Could you check a few things on this model? Use its own coordinates, in mm. Face numbers are marked on the shaded views. A direction names the side the tool comes from. Coordinates: 2 decimals unless noted, no trailing zeros. Loops run counter-clockwise (first coordinate to the right, second up) from the corner with the lowest first, then second, coordinate; pieces in that order, holes last.
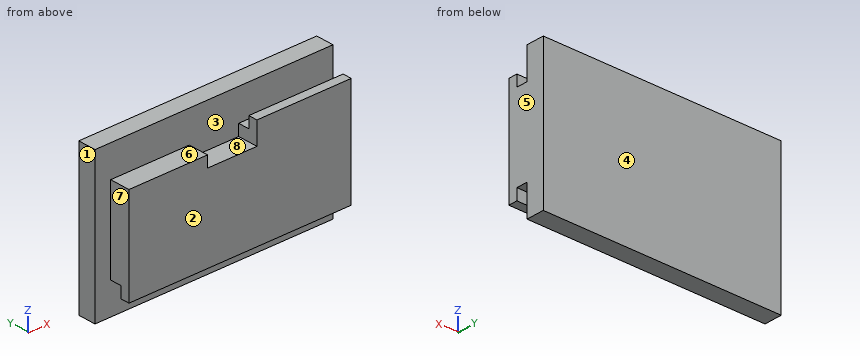
from build123d import *

# Parameters (mm, degrees)
F0_W     = 5.5
F0_H     = 4.5
F0_W_2   = 3.5
F0_H_2   = 2.5
F0_H_3   = 19
F0_W_3   = 11
F1_DEPTH = 4
F0_W_4   = 17.5
F0_W_5   = 46
F2_DEPTH = 8.5
F3_DEPTH = 1
F4_DEPTH = 6.5
F5_DEPTH = 4


with BuildPart() as f1:
    # F0 (on Front) → F1 (new body)
    with BuildSketch(Plane.XZ):
        Polygon((-23, -12), (-26.5, -12), (-26.5, -16.5), (26.5, -16.5), (26.5, -12), (23, -12), align=None)
        with Locations((-2.75, 14.25)):
            Rectangle(F0_W, F0_H)
        with Locations((2.75, 14.25)):
            Rectangle(F0_W, F0_H)
        Polygon((-5.5, 16.5), (-26.5, 16.5), (-26.5, 12), (-23, 12), (-5.5, 12), align=None)
        with Locations((-24.75, 10.75)):
            Rectangle(F0_W_2, F0_H_2)
        with Locations((-24.75, 0)):
            Rectangle(F0_W_2, F0_H_3)
        with Locations((-24.75, -10.75)):
            Rectangle(F0_W_2, F0_H_2)
        Polygon((0, 12), (-5.5, 12), (-5.5, 9.5), (5.5, 9.5), (5.5, 12), align=None)
        with Locations((0, 8.25)):
            Rectangle(F0_W_3, F0_H_2)
        Polygon((26.5, 16.5), (5.5, 16.5), (5.5, 12), (23, 12), (26.5, 12), align=None)
        with Locations((24.75, 10.75)):
            Rectangle(F0_W_2, F0_H_2)
        with Locations((24.75, 0)):
            Rectangle(F0_W_2, F0_H_3)
        with Locations((24.75, -10.75)):
            Rectangle(F0_W_2, F0_H_2)
    extrude(amount=F1_DEPTH)

    # F0 (on Front) → F2 (join)
    with BuildSketch(Plane.XZ):
        Polygon((-5.5, 7), (-5.5, 9.5), (-23, 9.5), (-23, -9.5), (23, -9.5), (23, 9.5), (5.5, 9.5), (5.5, 7), align=None)
        with Locations((14.25, 10.75)):
            Rectangle(F0_W_4, F0_H_2)
        with Locations((0, -10.75)):
            Rectangle(F0_W_5, F0_H_2)
        with Locations((24.75, 10.75)):
            Rectangle(F0_W_2, F0_H_2)
        with Locations((24.75, 0)):
            Rectangle(F0_W_2, F0_H_3)
        with Locations((24.75, -10.75)):
            Rectangle(F0_W_2, F0_H_2)
    extrude(amount=F2_DEPTH)

    # F0 (on Front) → F3 (join)
    with BuildSketch(Plane.XZ):
        with Locations((-2.75, 14.25)):
            Rectangle(F0_W, F0_H)
        with Locations((2.75, 14.25)):
            Rectangle(F0_W, F0_H)
    extrude(amount=F3_DEPTH)

    # F0 (on Front) → F4 (cut)
    with BuildSketch(Plane.XZ):
        with Locations((14.25, 10.75)):
            Rectangle(F0_W_4, F0_H_2)
        with Locations((0, -10.75)):
            Rectangle(F0_W_5, F0_H_2)
        with Locations((24.75, 10.75)):
            Rectangle(F0_W_2, F0_H_2)
        with Locations((24.75, -10.75)):
            Rectangle(F0_W_2, F0_H_2)
    extrude(amount=F4_DEPTH, mode=Mode.SUBTRACT)

    # F0 (on Front) → F5 (join)
    with BuildSketch(Plane.XZ):
        with Locations((14.25, 10.75)):
            Rectangle(F0_W_4, F0_H_2)
        with Locations((-14.25, 10.75)):
            Rectangle(F0_W_4, F0_H_2)
        with Locations((0, -10.75)):
            Rectangle(F0_W_5, F0_H_2)
        with Locations((24.75, 10.75)):
            Rectangle(F0_W_2, F0_H_2)
        with Locations((24.75, -10.75)):
            Rectangle(F0_W_2, F0_H_2)
    extrude(amount=F5_DEPTH)


solid = f1.part
1) Imagine slicing it at A-A on x = -4.5. List the corners of the cut face in (y, z) for me.
2) We'd pull the mould along Y, two halves only. Please class the marked faces 1, 2, 3 and 4: released by +Y, released by -Y, zero draft, split by the parting line, or undercut.
3) Imagine slicing it at B-B on y = -5. List the corners of the cut face in (x, z) for me.
4) For the marked faces 5, 6, 7 and 8, which set-ups out of +Z, -Z, +X, -X, +Y, -Y let a thin tool reach every point of the face, with its end or its side?
5) Imagine slicing it at D-D on x = 13.5. List the corners of the cut face in (y, z) for me, plus the area to 4 significant figures.
6) Imagine slicing it at C-C on z = -1. List the corners of the cut face in (x, y) for me, plus the area to 3 significant figures.
7) If I drill on L1, parallel to Y at x = 22, z = 10.5; L2, parallel to Y at x = -12.5, z = 13; L3, parallel to X at y = -5.25, z = -1, over which ranges is the centre line in solid material (lowest first)?
8) Will these pins go through, and if not, where does the flat tip stop? pin 1 (5 mm diameter, centred on y = -7, z = 0, fed in from -X); pin 2 (12 mm diameter, centred on x = -20, z = 11.5, fed in from -Y); pin 3 (3 mm diameter, centred on x = 18.5, y = -6, fed in from +Z); pin 4 (3.5 mm diameter, centred on x = -15.5, y = -6.5, fed in from +Z).
Solved:
1. outline: (-8.5, -12) - (-6.5, -12) - (-6.5, -9.5) - (-4, -9.5) - (-4, -16.5) - (0, -16.5) - (0, 16.5) - (-4, 16.5) - (-4, 7) - (-8.5, 7) - close
2. face 1: zero draft
2. face 2: released by -Y
2. face 3: undercut
2. face 4: released by +Y
3. outline: (-23, -9.5) - (26.5, -9.5) - (26.5, 9.5) - (5.5, 9.5) - (5.5, 7) - (-5.5, 7) - (-5.5, 9.5) - (-23, 9.5) - close
4. face 5: +Z, -Z, +X, +Y, -Y
4. face 6: +Z, -X, -Y
4. face 7: +Z, -Z, -X, -Y
4. face 8: +Z, -Y
5. outline: (-8.5, -12) - (-6.5, -12) - (-6.5, -9.5) - (-4, -9.5) - (-4, -16.5) - (0, -16.5) - (0, 16.5) - (-4, 16.5) - (-4, 9.5) - (-6.5, 9.5) - (-6.5, 12) - (-8.5, 12) - close
5. area: 227.5 mm2
6. outline: (-26.5, -4) - (-23, -4) - (-23, -8.5) - (26.5, -8.5) - (26.5, 0) - (-26.5, 0) - close
6. area: 435 mm2
7. L1: y = -8.5 to -6.5, -4 to 0
7. L2: y = -4 to 0
7. L3: x = -23 to 26.5
8. pin 1: stops at x = -23
8. pin 2: stops at y = -8.5
8. pin 3: stops at z = 12
8. pin 4: stops at z = 9.5
